Could you check a few things on this drawing? It's one solid part, dimensions in mm from its lowest x, y, z. Give positions to 0.01 mm unless a question says otherwise; leave off trailing zeros. Order: outer loops, then holes, each group sorted by start corner. A loop starts at its lowest first (then second) coordinate and runs counter-clockwise, first axis right, second up.
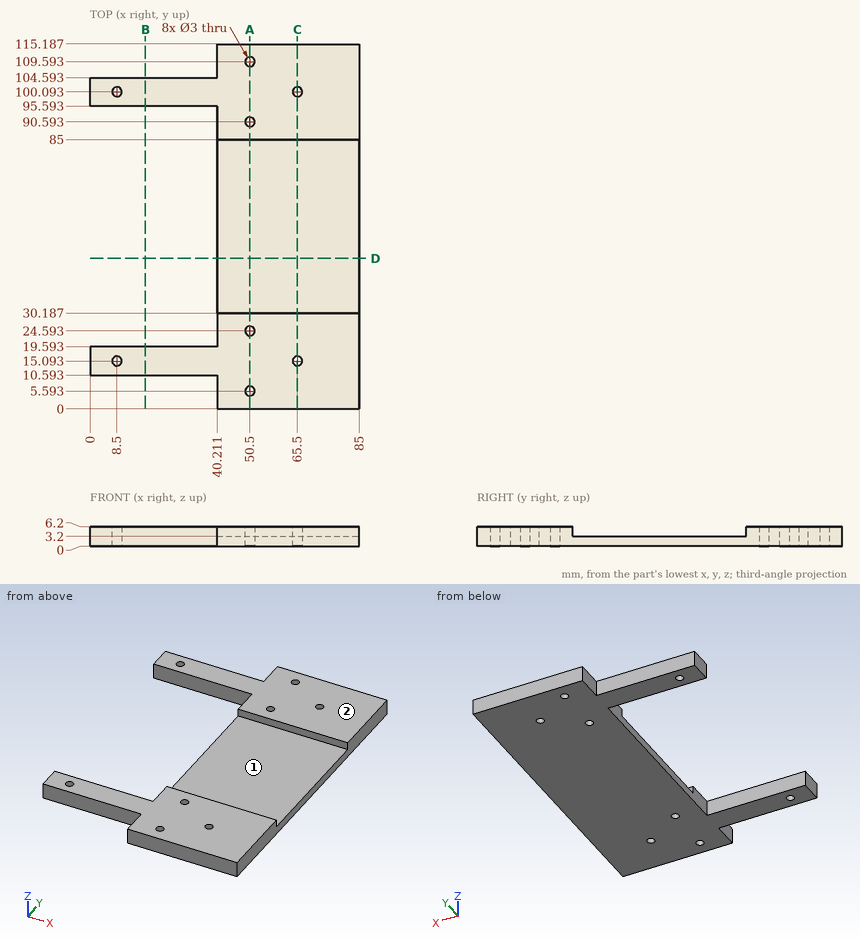
1) I'm going to push flat-ended pins straight in: pin 1 Ø2.5 at (x, y) = (50.5, 109.59) entering from -Z; pin 2 Ø1.9 at (x, z) = (28.5, 2) entering from -Y; pin 3 Ø1.5 at (y, z) = (26.5, 0.5) entering from -X; pin 4 Ø22.5 at (x, y) = (73.5, 48) entering from +Z. Where does each tip first touch, or does it pass through?
2) Suppose I cut it at C-C (x = 65.5). Please give me the cut outline in (y, z).
3) Suppose I cut it at A-A (x = 50.5). Please give me the cut outline in (y, z).
4) Suppose I cut it at D-D (y = 47.5). Please give me the cut outline in (x, z), and give its area (3 significant figures).
5) Suppose I cut it at B-B (x = 17.5). Please give me the cut outline in (y, z).
6) We'd pull the mould along Y, two halves only. Please class the marked faces 1 and 2: +Y half, -Y half, draft (parallel to the pull), parting line (faces both ways), or undercut.
7) If I drill on line 1 (Y direction, x = 65.5, z = 4); line 2 (Y direction, x = 18.5, z = 1.75); line 3 (Y direction, x = 77.5, z = 4.5), over which ranges is the centre line in solid material (lowest first)?
Results:
1. pin 1: passes through
1. pin 2: stops at y = 10.59
1. pin 3: stops at x = 40.21
1. pin 4: stops at z = 3.2
2. outline: (0, 0) - (13.59, 0) - (13.59, 6.2) - (0, 6.2) - close; (16.59, 0) - (98.59, 0) - (98.59, 6.2) - (85, 6.2) - (85, 3.2) - (30.19, 3.2) - (30.19, 6.2) - (16.59, 6.2) - close; (101.59, 0) - (115.19, 0) - (115.19, 6.2) - (101.59, 6.2) - close
3. outline: (0, 0) - (4.09, 0) - (4.09, 6.2) - (0, 6.2) - close; (7.09, 0) - (23.09, 0) - (23.09, 6.2) - (7.09, 6.2) - close; (26.09, 0) - (89.09, 0) - (89.09, 6.2) - (85, 6.2) - (85, 3.2) - (30.19, 3.2) - (30.19, 6.2) - (26.09, 6.2) - close; (92.09, 0) - (108.09, 0) - (108.09, 6.2) - (92.09, 6.2) - close; (111.09, 0) - (115.19, 0) - (115.19, 6.2) - (111.09, 6.2) - close
4. outline: (40.21, 0) - (85, 0) - (85, 3.2) - (40.21, 3.2) - close
4. area: 143 mm2
5. outline: (10.59, 0) - (19.59, 0) - (19.59, 6.2) - (10.59, 6.2) - close; (95.59, 0) - (104.59, 0) - (104.59, 6.2) - (95.59, 6.2) - close
6. face 1: undercut
6. face 2: draft
7. line 1: y = 0 to 13.59, 16.59 to 30.19, 85 to 98.59, 101.59 to 115.19
7. line 2: y = 10.59 to 19.59, 95.59 to 104.59
7. line 3: y = 0 to 30.19, 85 to 115.19
